Verification items for the finished model (mm, model axes). Face numbers are marked on the shaded views. A direction names the side the tool comes from. Give positions to 0.01 mm unless a question says otherwise; leave off trailing zeros. Write each loop counter-clockwise with the first axis right and the second up, starting at its lowest first coordinate (ties: lowest second). Pieces come first, ordered by that corner, then holes. Notation, with made-up numbers: M 16,-27 L 64,-27 A22 ccw 64,12 Z; hole C 86.25,-27.5 d5. An arc over 180 degrees is marked long. Write item = value, one per line.
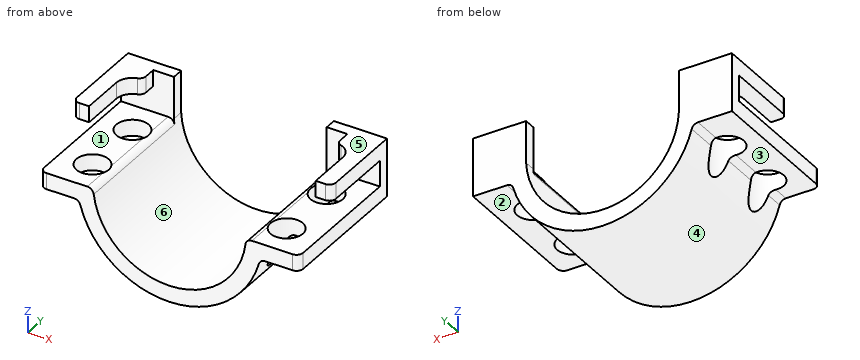
from build123d import *
from OCP.BRepAlgoAPI import BRepAlgoAPI_Cut
from OCP.TopTools import TopTools_ListOfShape

# Parameters (mm, degrees)
BOSS_EXTRUDE1_DEPTH = 27.94
SKETCH3_R           = 3.175
CUT_EXTRUDE1_DEPTH  = 53.100399864
BOSS_EXTRUDE2_START = -10.419367
BOSS_EXTRUDE2_DEPTH = 10.419367
CUT_EXTRUDE2_DEPTH  = 6.35
FILLET1_R           = 1.27


with BuildPart() as part:
    # Sketch2 → Boss-Extrude1 (new body)
    with BuildSketch(Plane(origin=(0, 0, 0), x_dir=(1, 0, 0), z_dir=(0, 1, 0))):
        with BuildLine():
            Line((0, 0), (-10.419367303, 0))
            Line((-10.419367303, 0), (-10.419367303, 3.175))
            Line((-10.419367303, 3.175), (-2.762835284, 3.175))
            ThreePointArc((-2.762835284, 3.175), (14.980632697, 17.413), (32.724100678, 3.175))
            Line((32.724100678, 3.175), (40.380632697, 3.175))
            Line((40.380632697, 3.175), (40.380632697, 0))
            Line((40.380632697, 0), (29.961265394, 0))
            ThreePointArc((29.961265394, 0), (14.980632697, 14.238), (0, 0))
        make_face()
    extrude(amount=-BOSS_EXTRUDE1_DEPTH)

    # Sketch3 → Cut-Extrude1 (cut, through all)
    with BuildSketch(Plane.XY):
        with Locations((-4.069367303, -8.89)):
            Circle(SKETCH3_R)
        with Locations((34.030632697, -8.89)):
            Circle(SKETCH3_R)
        with Locations((-4.069367303, -21.59)):
            Circle(SKETCH3_R)
        with Locations((34.030632697, -21.59)):
            Circle(SKETCH3_R)
    extrude(amount=-CUT_EXTRUDE1_DEPTH, mode=Mode.SUBTRACT)

    # Sketch4 → Boss-Extrude2 (add)
    with BuildSketch(Plane(origin=(40.380632697, 0, 0), x_dir=(0, 0, -1), z_dir=(1, 0, 0)).offset(BOSS_EXTRUDE2_START)):
        Polygon((-5.08, -17.526), (-8.255, -17.526), (-8.255, 0), (0, 0), (0, -2.286), (-5.08, -2.286), align=None)
    boss_extrude2 = extrude(amount=BOSS_EXTRUDE2_DEPTH)


with BuildPart() as cut_extrude2_tool:
    # Sketch5 → Cut-Extrude2 (new body)
    with BuildSketch(Plane.XY.offset(8.255)):
        with BuildLine():
            Line((37.205632697, -8.89), (37.205632697, -17.526))
            Line((37.205632697, -17.526), (29.961265394, -17.526))
            Line((29.961265394, -17.526), (29.961265394, -2.286))
            Line((29.961265394, -2.286), (34.030632697, -2.286))
            Line((34.030632697, -2.286), (34.030632697, -5.715))
            ThreePointArc((34.030632697, -5.715), (36.275696727, -6.64493597), (37.205632697, -8.89))
        make_face()
    cut_extrude2 = extrude(amount=-CUT_EXTRUDE2_DEPTH)


with BuildPart() as part_1:
    add(part.part)

    # Cut-Extrude2: cut by cut_extrude2_tool, with a tolerance
    cut_extrude2_stock = TopTools_ListOfShape()
    cut_extrude2_stock.Append(part_1.part.wrapped)
    cut_extrude2_tools = TopTools_ListOfShape()
    cut_extrude2_tools.Append(cut_extrude2_tool.part.wrapped)
    cut_extrude2_cut = BRepAlgoAPI_Cut()
    cut_extrude2_cut.SetArguments(cut_extrude2_stock)
    cut_extrude2_cut.SetTools(cut_extrude2_tools)
    cut_extrude2_cut.SetFuzzyValue(0.00001)
    cut_extrude2_cut.Build()
    add(Compound.cast(cut_extrude2_cut.Shape()).solids(), mode=Mode.REPLACE)

    # Mirror1: Boss-Extrude2, Cut-Extrude2 across plane
    add(boss_extrude2.mirror(Plane.ZY.offset(-14.980632697)))
    add(cut_extrude2.mirror(Plane.ZY.offset(-14.980632697)), mode=Mode.SUBTRACT)

    # Fillet1
    # the kernel refuses this fillet: 1.27 mm, written as the material it adds along each edge
    with BuildSketch(Plane(origin=(32.724100678, 0, -3.175), x_dir=(1, 0, 0), z_dir=(0, -1, 0))) as fillet1_piece_1_section:
        with BuildLine():
            CenterArc((0.991397271, -1.27), FILLET1_R, 90, 74.467738735)
            ThreePointArc((-0.232222111, -0.929918231), (-0.109979978, -0.466490187), (0, 0))
            Line((0, 0), (0.991397271, 0))
        make_face()
    fillet1_piece_1 = extrude(amount=8.474776002, mode=Mode.PRIVATE)
    fillet1_piece_1 = fillet1_piece_1 - Plane(origin=(34.030632697, -8.89, -3.175), x_dir=(1, 0, 0), z_dir=(0, 0, 1)) * Cylinder(3.175, 21, mode=Mode.PRIVATE)
    add(fillet1_piece_1)
    with BuildSketch(Plane(origin=(32.724100678, -22.005223998, -3.175), x_dir=(1, 0, 0), z_dir=(0, -1, 0))) as fillet1_piece_2_section:
        with BuildLine():
            CenterArc((0.991397271, -1.27), FILLET1_R, 90, 74.467738735)
            ThreePointArc((-0.232222111, -0.929918231), (-0.109979978, -0.466490187), (0, 0))
            Line((0, 0), (0.991397271, 0))
        make_face()
    fillet1_piece_2 = extrude(amount=5.934776002, mode=Mode.PRIVATE)
    fillet1_piece_2 = fillet1_piece_2 - Plane(origin=(34.030632697, -21.59, -3.175), x_dir=(1, 0, 0), z_dir=(0, 0, 1)) * Cylinder(3.175, 16, mode=Mode.PRIVATE)
    add(fillet1_piece_2)
    with BuildSketch(Plane(origin=(32.724100678, -9.305223998, -3.175), x_dir=(1, 0, 0), z_dir=(0, -1, 0))) as fillet1_piece_3_section:
        with BuildLine():
            CenterArc((0.991397271, -1.27), FILLET1_R, 90, 74.467738735)
            ThreePointArc((-0.232222111, -0.929918231), (-0.109979978, -0.466490187), (0, 0))
            Line((0, 0), (0.991397271, 0))
        make_face()
    fillet1_piece_3 = extrude(amount=11.869552004, mode=Mode.PRIVATE)
    fillet1_piece_3 = fillet1_piece_3 - Plane(origin=(34.030632697, -21.59, -3.175), x_dir=(1, 0, 0), z_dir=(0, 0, 1)) * Cylinder(3.175, 28, mode=Mode.PRIVATE)
    fillet1_piece_3 = fillet1_piece_3 - Plane(origin=(34.030632697, -8.89, -3.175), x_dir=(1, 0, 0), z_dir=(0, 0, 1)) * Cylinder(3.175, 28, mode=Mode.PRIVATE)
    add(fillet1_piece_3)
    with BuildSketch(Plane(origin=(-2.762835284, 0, -3.175), x_dir=(0.24228281636804117, 0, -0.9702056673163532), z_dir=(0, -1, 0))) as fillet1_piece_4_section:
        with BuildLine():
            CenterArc((0.991962675, -1.269558427), FILLET1_R, 91.510947972, 74.467738735)
            Line((-0.240198523, -0.96185925), (0, 0))
            ThreePointArc((0, 0), (0.479237682, -0.006319359), (0.958475365, 0))
        make_face()
    fillet1_piece_4 = extrude(amount=8.474776002, mode=Mode.PRIVATE)
    fillet1_piece_4 = fillet1_piece_4 - Plane(origin=(-4.069367303, -8.89, -3.175), x_dir=(1, 0, 0), z_dir=(0, 0, 1)) * Cylinder(3.175, 21, mode=Mode.PRIVATE)
    add(fillet1_piece_4)
    with BuildSketch(Plane(origin=(-2.762835284, -22.005223998, -3.175), x_dir=(0.24228281636804117, 0, -0.9702056673163532), z_dir=(0, -1, 0))) as fillet1_piece_5_section:
        with BuildLine():
            CenterArc((0.991962675, -1.269558427), FILLET1_R, 91.510947972, 74.467738735)
            Line((-0.240198523, -0.96185925), (0, 0))
            ThreePointArc((0, 0), (0.479237682, -0.006319359), (0.958475365, 0))
        make_face()
    fillet1_piece_5 = extrude(amount=5.934776002, mode=Mode.PRIVATE)
    fillet1_piece_5 = fillet1_piece_5 - Plane(origin=(-4.069367303, -21.59, -3.175), x_dir=(1, 0, 0), z_dir=(0, 0, 1)) * Cylinder(3.175, 16, mode=Mode.PRIVATE)
    add(fillet1_piece_5)
    with BuildSketch(Plane(origin=(-2.762835284, -9.305223998, -3.175), x_dir=(0.24228281636804117, 0, -0.9702056673163532), z_dir=(0, -1, 0))) as fillet1_piece_6_section:
        with BuildLine():
            CenterArc((0.991962675, -1.269558427), FILLET1_R, 91.510947972, 74.467738735)
            Line((-0.240198523, -0.96185925), (0, 0))
            ThreePointArc((0, 0), (0.479237682, -0.006319359), (0.958475365, 0))
        make_face()
    fillet1_piece_6 = extrude(amount=11.869552004, mode=Mode.PRIVATE)
    fillet1_piece_6 = fillet1_piece_6 - Plane(origin=(-4.069367303, -21.59, -3.175), x_dir=(1, 0, 0), z_dir=(0, 0, 1)) * Cylinder(3.175, 28, mode=Mode.PRIVATE)
    fillet1_piece_6 = fillet1_piece_6 - Plane(origin=(-4.069367303, -8.89, -3.175), x_dir=(1, 0, 0), z_dir=(0, 0, 1)) * Cylinder(3.175, 28, mode=Mode.PRIVATE)
    add(fillet1_piece_6)
    # the kernel refuses this fillet: 1.27 mm, written as the material it takes off along each edge
    with BuildSketch(Plane(origin=(29.961265394, 2.904944682, 0), x_dir=(-0.08790703364756058, 0, -0.9961286831706467), z_dir=(0, -1, 0))) as fillet1_2_piece_1_section:
        with BuildLine():
            CenterArc((1.1629374, 1.269121421), FILLET1_R, 185.043211655, 82.825455624)
            Line((-0.102146028, 1.157479488), (0, 0))
            ThreePointArc((0, 0), (0.557852926, 0.010376919), (1.115705852, 0))
        make_face()
    fillet1_2_piece_1 = extrude(amount=33.749889363, mode=Mode.PRIVATE)
    fillet1_2_piece_1 = split(fillet1_2_piece_1, bisect_by=Plane(origin=(29.961265394, -2.286, 0), z_dir=(0, -1, 0)), keep=Keep.TOP, mode=Mode.PRIVATE)
    add(fillet1_2_piece_1, mode=Mode.SUBTRACT)
    with BuildSketch(Plane(origin=(0, 2.904944682, 0), x_dir=(-1, 0, 0), z_dir=(0, -1, 0))) as fillet1_2_piece_2_section:
        with BuildLine():
            CenterArc((1.161977873, 1.27), FILLET1_R, 187.174544376, 82.825455624)
            ThreePointArc((-0.098078392, 1.111386601), (-0.038702449, 0.556605505), (0, 0))
            Line((0, 0), (1.161977873, 0))
        make_face()
    fillet1_2_piece_2 = extrude(amount=33.749889363, mode=Mode.PRIVATE)
    fillet1_2_piece_2 = split(fillet1_2_piece_2, bisect_by=Plane(origin=(0, -2.286, 0), z_dir=(0, -1, 0)), keep=Keep.TOP, mode=Mode.PRIVATE)
    add(fillet1_2_piece_2, mode=Mode.SUBTRACT)
    with BuildSketch(Plane(origin=(-10.419367303, -17.526, 1.905), x_dir=(0, 1, 0), z_dir=(0, 0, 1)), Plane(origin=(40.380632697, -27.94, -6.35), x_dir=(-1, 0, 0), z_dir=(0, 0, 1)), Plane(origin=(40.380632697, -17.526, 1.905), x_dir=(-1, 0, 0), z_dir=(0, 0, 1))) as fillet1_2_piece_3:
        with BuildLine():
            CenterArc((FILLET1_R, -FILLET1_R), FILLET1_R, 90, 90)
            Line((0, -FILLET1_R), (0, 0))
            Line((0, 0), (FILLET1_R, 0))
        make_face()
    extrude(amount=9.525, mode=Mode.SUBTRACT)
    with BuildSketch(Plane(origin=(-10.419367303, -27.94, 3.175), x_dir=(0, 1, 0), z_dir=(0, 0, -1))) as fillet1_2_piece_4:
        with BuildLine():
            CenterArc((FILLET1_R, FILLET1_R), FILLET1_R, 180, 90)
            Line((0, FILLET1_R), (0, 0))
            Line((0, 0), (FILLET1_R, 0))
        make_face()
    extrude(amount=9.525, mode=Mode.SUBTRACT)
    with BuildSketch(Plane(origin=(34.030632697, -5.715, 10.966773743), x_dir=(0, 1, 0), z_dir=(0, 0, -1))) as fillet1_2_piece_5:
        with BuildLine():
            CenterArc((1.084709497, 1.27), FILLET1_R, 196.601549599, 73.398450401)
            ThreePointArc((-0.132350359, 0.907142857), (-0.033261818, 0.458373423), (0, 0))
            Line((0, 0), (1.084709497, 0))
        make_face()
    extrude(amount=8.598547486, mode=Mode.SUBTRACT)
    with BuildSketch(Plane(origin=(-4.069367303, -5.715, 10.966773743), x_dir=(0, 1, 0), z_dir=(0, 0, -1))) as fillet1_2_piece_6:
        with BuildLine():
            CenterArc((1.084709497, -1.27), FILLET1_R, 90, 73.398450401)
            ThreePointArc((-0.132350359, -0.907142857), (-0.033261818, -0.458373423), (0, 0))
            Line((0, 0), (1.084709497, 0))
        make_face()
    extrude(amount=8.598547486, mode=Mode.SUBTRACT)


solid = part_1.part
1) Cross-section at B-B on y = -21.59. Record the boundary of the cut face in (x, z) (3 decimals).
From the geometry:
outline = M -10.419,-3.175 L -7.244,-3.175 L -7.244,0 L -10.419,0 Z; M -0.894,-8.088 A18.175 ccw 30.856,-8.088 L 30.856,-0.029 A1.27 ccw 29.863,-1.111 A15 cw 0.098,-1.111 A1.27 ccw -0.894,-0.029 Z; M 37.206,-3.175 L 40.381,-3.175 L 40.381,0 L 37.206,0 Z
2) Cross-section at C-C on z = -13.5. Record the boundary of the cut face in (x, y), plus the area to 3 significant figures.
From the geometry:
outline = M 3.71,-27.94 L 10.33,-27.94 L 10.33,0 L 3.71,0 Z; M 19.63,-27.94 L 26.25,-27.94 L 26.25,0 L 19.63,0 Z
area = 370 mm^2
3) Draft check along X on the marked faces 4, 5 and 6. Enter one of: +X half, -X half, draft (parallel to the pull), parting line (faces both ways), or undercut.
From the geometry:
face_4 = parting line
face_5 = draft
face_6 = undercut
4) Cross-section at D-D on x = 3. Record the boundary of the cut face in (y, z), plus the area to 3 significant figures.
From the geometry:
outline = M -27.94,-12.91 L 0,-12.91 L 0,-8.26 L -27.94,-8.26 Z
area = 130 mm^2
5) Cross-section at A-A on z = 4.5. Record the boundary of the cut face in (x, y).
From the geometry:
outline = M -10.42,-2.29 L 0,-2.29 L 0,0 L -10.42,0 Z; M 29.96,-2.29 L 40.38,-2.29 L 40.38,0 L 29.96,0 Z
6) Depth check by flat-ended pin: P1, Ø3, axis at x = 4.5, y = -8.5, coming from the +Z side; P2, Ø7.5, axis at x = 37.5, y = -16.5, coming from the -Z side (3 decimals); P3, Ø1, axis at x = -8, z = 6.5, coming from the -Y side. Enter the tip coordinate at first touch or a pass-through.
From the geometry:
P1 = -8.26
P2 = -3.175
P3 = -17.53
7) Tool access check on the marked faces 1, 2 and 3. Record the directions out of +Z, -Z, +X, -X, +Y, -Y that give a thin tool (end or side, any length) a straight path to the whole face; none if there is none.
From the geometry:
face_1 = +X, -X, -Y
face_2 = -Z, +X, +Y, -Y
face_3 = -Z, -X, +Y, -Y
8) Material ranges on probe 1 along X at (y, z) = (-22, -1.5); probe 2 along X at (y, z) = (-10.75, -1.25); probe 3 along Y at (x, z) = (30.5, 3.25), recorded low to high. Write a range as from..to.
From the geometry:
probe_1 = -10.42..-7.22, -0.92..0.15, 29.81..30.88, 37.18..40.38
probe_2 = -10.42..-6.64, -1.5..0.12, 29.85..31.46, 36.6..40.38
probe_3 = -2.29..0
